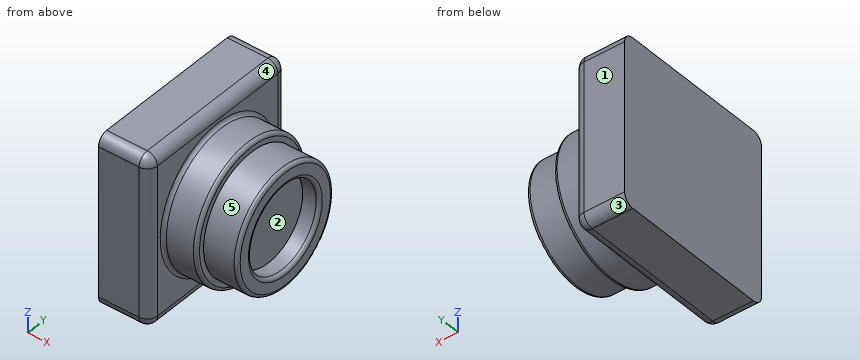
from build123d import *

# Parameters (mm, degrees)
SKETCH1_W           = 50
SKETCH1_H           = 50
BOSS_EXTRUDE1_DEPTH = 15
SKETCH2_R           = 20
BOSS_EXTRUDE2_DEPTH = 20
CUT_EXTRUDE1_START  = -10
SKETCH3_R           = 20
SKETCH3_R_2         = 17.5
SKETCH3_R_3         = 12.5
CUT_EXTRUDE1_DEPTH  = 10
SKETCH4_R           = 12.5
BOSS_EXTRUDE3_DEPTH = 5
FILLET1_R           = 1
FILLET2_R           = 3
FILLET3_R           = 3


with BuildPart() as part:
    # Sketch1 → Boss-Extrude1 (new body)
    with BuildSketch(Plane(origin=(0, 0, 0), x_dir=(0, 0, -1), z_dir=(1, 0, 0))):
        Rectangle(SKETCH1_W, SKETCH1_H)
    extrude(amount=BOSS_EXTRUDE1_DEPTH)

    # Sketch2 → Boss-Extrude2 (add)
    with BuildSketch(Plane(origin=(15, 0, 0), x_dir=(0, 0, -1), z_dir=(1, 0, 0))):
        Circle(SKETCH2_R)
    extrude(amount=BOSS_EXTRUDE2_DEPTH)

    # Sketch3 → Cut-Extrude1 (cut)
    # profile 1 of 2: a face of its own
    with BuildSketch(Plane(origin=(35, 0, 0), x_dir=(0, 0, -1), z_dir=(1, 0, 0)).offset(CUT_EXTRUDE1_START)):
        Circle(SKETCH3_R)
        Circle(SKETCH3_R_2, mode=Mode.SUBTRACT)
    # profile 2 of 2: a face of its own
    with BuildSketch(Plane(origin=(35, 0, 0), x_dir=(0, 0, -1), z_dir=(1, 0, 0)).offset(CUT_EXTRUDE1_START)):
        Circle(SKETCH3_R_3)
    extrude(amount=CUT_EXTRUDE1_DEPTH, mode=Mode.SUBTRACT)

    # Sketch4 → Boss-Extrude3 (add)
    with BuildSketch(Plane(origin=(25, 0, 0), x_dir=(0, 0, -1), z_dir=(1, 0, 0))):
        Circle(SKETCH4_R)
    extrude(amount=BOSS_EXTRUDE3_DEPTH)

    # Fillet1
    fillet1_edges = [part.edges().sort_by_distance(p)[0] for p in [
        (15, 0, 20),
        (35, 0, 12.5),
        (35, 0, 17.5),
        (25, 0, 20),
    ]]
    fillet(fillet1_edges, radius=FILLET1_R)

    # Fillet2
    fillet2_edges = [part.edges().sort_by_distance(p)[0] for p in [
        (15, 0, 25),
        (15, -25, 0),
        (15, 0, -25),
        (15, 25, 0),
    ]]
    fillet(fillet2_edges, radius=FILLET2_R)

    # Fillet3
    # the kernel refuses this fillet: 3 mm, written as the material it takes off along each edge
    with BuildSketch(Plane(origin=(12, 22, 22), x_dir=(0, 1, 0), z_dir=(0, 0, 1))) as fillet3_piece_1_section:
        Polygon((0, 0), (FILLET3_R, 0), (FILLET3_R, -FILLET3_R), (0, -FILLET3_R), align=None)
    fillet3_piece_1 = extrude(amount=FILLET3_R, mode=Mode.PRIVATE)
    fillet3_piece_1 = fillet3_piece_1 - Plane(origin=(12, 22, 22), x_dir=(-0.7071067811865475, -0.7071067811865475, 0), z_dir=(0, 0, 1)) * Sphere(FILLET3_R, mode=Mode.PRIVATE)
    add(fillet3_piece_1, mode=Mode.SUBTRACT)
    with BuildSketch(Plane(origin=(12, 22, -22), x_dir=(0, 0, -1), z_dir=(0, 1, 0))) as fillet3_piece_2_section:
        Polygon((0, 0), (FILLET3_R, 0), (FILLET3_R, -FILLET3_R), (0, -FILLET3_R), align=None)
    fillet3_piece_2 = extrude(amount=FILLET3_R, mode=Mode.PRIVATE)
    fillet3_piece_2 = fillet3_piece_2 - Plane(origin=(12, 22, -22), x_dir=(-0.7071067811865475, 0, 0.7071067811865475), z_dir=(0, 1, 0)) * Sphere(FILLET3_R, mode=Mode.PRIVATE)
    add(fillet3_piece_2, mode=Mode.SUBTRACT)
    with BuildSketch(Plane(origin=(12, -22, 22), x_dir=(0, -1, 0), z_dir=(0, 0, 1))) as fillet3_piece_3_section:
        Polygon((0, 0), (FILLET3_R, 0), (FILLET3_R, FILLET3_R), (0, FILLET3_R), align=None)
    fillet3_piece_3 = extrude(amount=FILLET3_R, mode=Mode.PRIVATE)
    fillet3_piece_3 = fillet3_piece_3 - Plane(origin=(12, -22, 22), x_dir=(-0.7071067811865475, 0.7071067811865475, 0), z_dir=(0, 0, 1)) * Sphere(FILLET3_R, mode=Mode.PRIVATE)
    add(fillet3_piece_3, mode=Mode.SUBTRACT)
    with BuildSketch(Plane(origin=(12, -22, -22), x_dir=(0, 0, -1), z_dir=(0, -1, 0))) as fillet3_piece_4_section:
        Polygon((0, 0), (FILLET3_R, 0), (FILLET3_R, FILLET3_R), (0, FILLET3_R), align=None)
    fillet3_piece_4 = extrude(amount=FILLET3_R, mode=Mode.PRIVATE)
    fillet3_piece_4 = fillet3_piece_4 - Plane(origin=(12, -22, -22), x_dir=(-0.7071067811865475, 0, 0.7071067811865475), z_dir=(0, -1, 0)) * Sphere(FILLET3_R, mode=Mode.PRIVATE)
    add(fillet3_piece_4, mode=Mode.SUBTRACT)
    with BuildSketch(Plane(origin=(-7.5, -25, -25), x_dir=(0, 0, 1), z_dir=(1, 0, 0)), Plane(origin=(-7.5, -25, 25), x_dir=(0, 1, 0), z_dir=(1, 0, 0))) as fillet3_piece_5:
        with BuildLine():
            CenterArc((FILLET3_R, -FILLET3_R), FILLET3_R, 90, 90)
            Line((0, -FILLET3_R), (0, 0))
            Line((0, 0), (FILLET3_R, 0))
        make_face()
    extrude(amount=19.5, mode=Mode.SUBTRACT)
    with BuildSketch(Plane(origin=(-7.5, 25, -25), x_dir=(0, 0, 1), z_dir=(1, 0, 0)), Plane(origin=(-7.5, 25, 25), x_dir=(0, -1, 0), z_dir=(1, 0, 0))) as fillet3_piece_6:
        with BuildLine():
            CenterArc((FILLET3_R, FILLET3_R), FILLET3_R, 180, 90)
            Line((0, FILLET3_R), (0, 0))
            Line((0, 0), (FILLET3_R, 0))
        make_face()
    extrude(amount=19.5, mode=Mode.SUBTRACT)


solid = part.part
Design review of the part built by this model. Coordinates are the model's own, in mm. Face numbers are marked on the shaded views. A direction names the side the tool comes from. Round coordinates to 2 decimals unless told otherwise and drop trailing zeros. Write each loop counter-clockwise with the first axis right and the second up, starting at its lowest first coordinate (ties: lowest second). Pieces come first, ordered by that corner, then holes.
Item 1: Draft analysis for pull direction Z (two halves, no side actions). For the marked faces 1, 2 and 3, state which applies: released by +Z, released by -Z, zero draft, split by the parting line, or undercut.
Item 2: Wall thickness on L1, parallel to Y at x = 32.75, z = 0; L2, parallel to X at y = 22, z = -15.5; L3, parallel to X at y = -6, z = 2: over which ranges is each line inside the solid? List them lowest first.
Item 3: For the marked faces 4 and 5, list the 3-axis set-ups (+Z, -Z, +X, -X, +Y, -Y) from which the entire face can be reached by the end or side of a thin tool; tool diameter is ignored.
Item 4: Consider section D-D on x = 21. Give the boundary of the cut face in (y, z).
Item 5: Consider section C-C on x = 33. Give the boundary of the cut face in (y, z), and give its area (3 significant figures).
Item 6: For pin 1 Ø2 at (x, y) = (25, -18) entering from +Z; pin 2 Ø1 at (x, z) = (18, 7.5) entering from +Y (3 decimals); pin 3 Ø1.5 at (x, y) = (28.5, 13) entering from +Z, all flat-tipped, find the tip position at first contact; note any pin that passes through.
Item 7: Consider section A-A on y = 0. Give the boundary of the cut face in (x, z).
Check values:
1. face 1: zero draft
1. face 2: undercut
1. face 3: released by -Z
2. L1: y = -17.5 to -12.5, 12.5 to 17.5
2. L2: x = 0 to 15
2. L3: x = 0 to 30
3. face 4: +Z, +X, +Y, -Y
3. face 5: +X
4. outline: circle Ø40 at (0, 0)
5. outline: circle Ø35 at (0, 0); hole circle Ø25 at (0, 0)
5. area: 471 mm2
6. pin 1: stops at z = 10.06
6. pin 2: stops at y = 18.735
6. pin 3: stops at z = 12.5
7. outline: (0, -25) - (12, -25) arc R3 ccw to (15, -22) - (15, -21) arc R1 cw to (16, -20) - (24, -20) arc R1 ccw to (25, -19) - (25, -17.5) - (34, -17.5) arc R1 ccw to (35, -16.5) - (35, -13.5) arc R1 ccw to (34, -12.5) - (30, -12.5) - (30, 12.5) - (34, 12.5) arc R1 ccw to (35, 13.5) - (35, 16.5) arc R1 ccw to (34, 17.5) - (25, 17.5) - (25, 19) arc R1 ccw to (24, 20) - (16, 20) arc R1 cw to (15, 21) - (15, 22) arc R3 ccw to (12, 25) - (0, 25) - close
